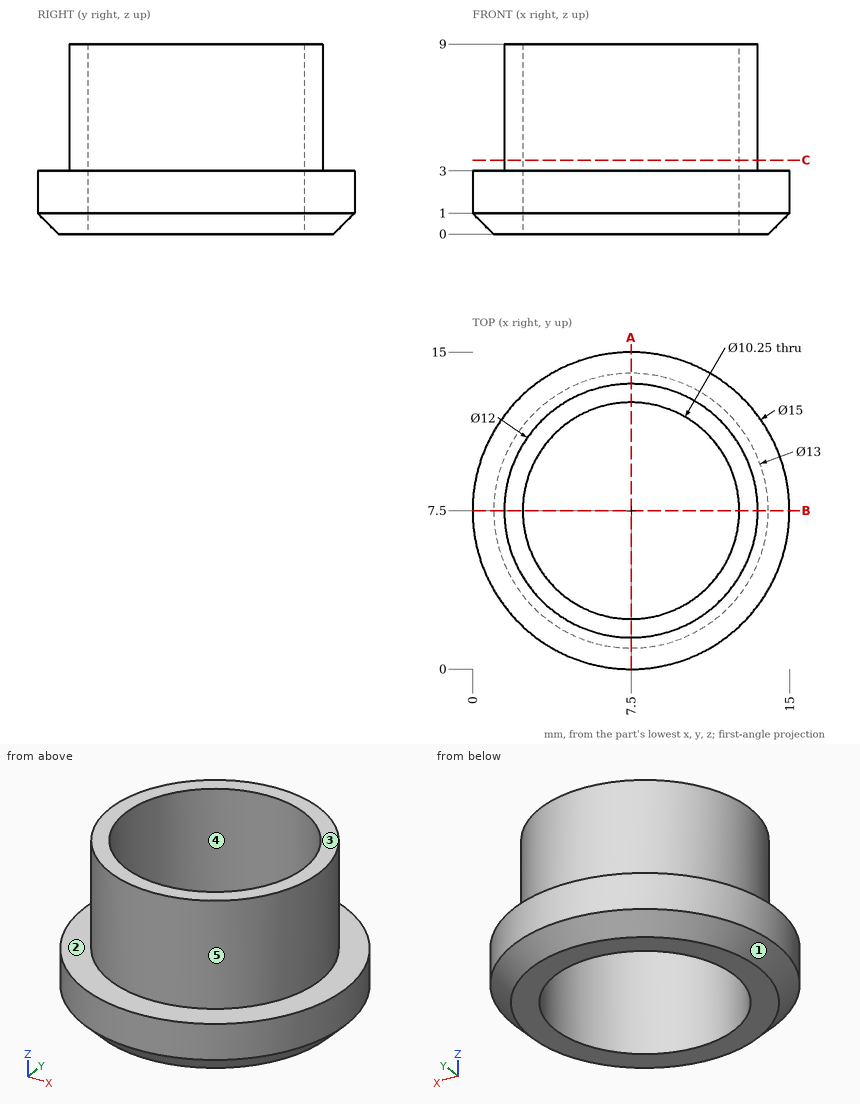
Design review of the part shown in the three views and the two pictorial views. Dimensions are in mm from the part's minimum x, y and z. A direction names the side the tool comes from. Round coordinates to 2 decimals unless told otherwise and drop trailing zeros. Write each loop counter-clockwise with the first axis right and the second up, starting at its lowest first coordinate (ties: lowest second). Pieces come first, ordered by that corner, then holes.
Item 1: Consider section A-A on x = 7.5. Give the boundary of the cut face in (y, z) (3 decimals), and give its area (4 significant figures).
Item 2: For the marked faces 1 and 2, list the 3-axis set-ups (+Z, -Z, +X, -X, +Y, -Y) from which the entire face can be reached by the end or side of a thin tool; tool diameter is ignored.
Item 3: Draft analysis for pull direction X (two halves, no side actions). For the marked faces 3, 4 and 5, state which applies: released by +X, released by -X, zero draft, split by the parting line, or undercut.
Item 4: Wall thickness on L1, parallel to Y at x = 7.5, z = 3.5 (3 decimals); L2, parallel to Y at x = 7.5, z = 2 (3 decimals); L3, parallel to Z at x = 1.75, y = 5.5: over which ranges is each line inside the solid? List them lowest first.
Item 5: Consider section C-C on z = 3.5. Give the boundary of the cut face in (x, y) (3 decimals), and give its area (3 significant figures).
Item 6: For pin 1 Ø2 at (y, z) = (12.5, 3.5) entering from -X; pin 2 Ø7.5 at (x, y) = (10, 7) entering from +Z; pin 3 Ø5 at (x, z) = (13.5, 6.5) entering from +Y, all flat-tipped, find the tip position at first contact; note any pin that passes through.
Check values:
1. outline: (0, 1) - (1, 0) - (2.375, 0) - (2.375, 9) - (1.5, 9) - (1.5, 3) - (0, 3) - close; (12.625, 0) - (14, 0) - (15, 1) - (15, 3) - (13.5, 3) - (13.5, 9) - (12.625, 9) - close
1. area: 23.75 mm2
2. face 1: -Z
2. face 2: +Z
3. face 3: zero draft
3. face 4: undercut
3. face 5: split by the parting line
4. L1: y = 1.5 to 2.375, 12.625 to 13.5
4. L2: y = 0 to 2.375, 12.625 to 15
4. L3: z = 0 to 3
5. outline: circle Ø12 at (7.5, 7.5); hole circle Ø10.25 at (7.5, 7.5)
5. area: 30.6 mm2
6. pin 1: stops at x = 1.24
6. pin 2: stops at z = 9
6. pin 3: stops at y = 12.37
